CAD build for the part. Positions are in the model's coordinates, mm. Give positions to 0.01 mm unless a question says otherwise; leave off trailing zeros. Order: outer loops, then holes, each group sorted by start corner. A loop starts at its lowest first (then second) coordinate and runs counter-clockwise, first axis right, second up.
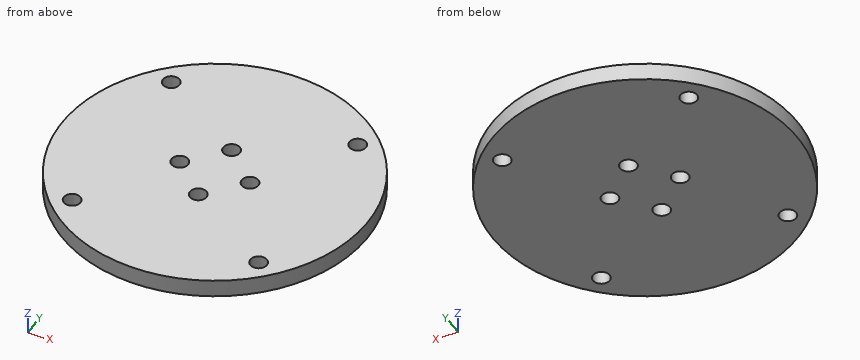
Solid Edge part; units mm, degrees
sketch "Sketch1" plane through (0, 0, 0) normal (0, 0, 1) x (1, 0, 0)
  circle A0 centre (0, 0) radius 31.0025
  circle A1 centre (19.0229, 19.0229) radius 1.7
  circle A2 centre (19.0229, -19.0229) radius 1.7
  circle A3 centre (-19.0229, -19.0229) radius 1.7
  circle A4 centre (-19.0229, 19.0229) radius 1.7
  circle A5 centre (-0.3206, 6.9927) radius 1.7
  circle A6 centre (6.9927, 0.3206) radius 1.7
  circle A7 centre (0.3206, -6.9927) radius 1.7
  circle A8 centre (-6.9927, -0.3206) radius 1.7
extrude "Protrusion1" add sketch "Sketch1" along normal blind 3.6
1. Saw through at C-C on z = 2.6. State how many separate pieces and enclosed holes the cut face has, plus the area to 3 significant figures.
2. Saw through at B-B on x = 0. Give the cut face in (y, z).
3. Wall check: line 1 (X direction, y = 1, z = 0.75); line 2 (X direction, y = -18, z = 3); line 3 (Y direction, x = 18.5, z = 1.7). Give the ranges that are in metal, low to high.
4. Saw through at A-A on x = -7. Give the cut face in (y, z).
5. Pin check, flat tips, straight feed: P1, Ø2, axis at x = 0.32, y = -6.99, coming from the +Z side; P2, Ø1, axis at x = 0.5, z = 1, coming from the +Y side. Stop position of each tip, or through.
6. Saw through at D-D on y = 25.5. Give the cut face in (x, z).
Reported:
1. separate pieces: 1
1. enclosed holes: 8
1. area: 2,950 mm2
2. outline: (-31, 0) - (-8.66, 0) - (-8.66, 3.6) - (-31, 3.6) - close; (-5.32, 0) - (5.32, 0) - (5.32, 3.6) - (-5.32, 3.6) - close; (8.66, 0) - (31, 0) - (31, 3.6) - (8.66, 3.6) - close
3. line 1: x = -30.99 to -8.06, -5.92 to 5.43, 8.55 to 30.99
3. line 2: x = -25.24 to -20.38, -17.67 to 17.67, 20.38 to 25.24
3. line 3: y = -24.88 to -20.64, -17.41 to 17.41, 20.64 to 24.88
4. outline: (-30.2, 0) - (-2.02, 0) - (-2.02, 3.6) - (-30.2, 3.6) - close; (1.38, 0) - (30.2, 0) - (30.2, 3.6) - (1.38, 3.6) - close
5. P1: passes through
5. P2: stops at y = 31
6. outline: (-17.63, 0) - (17.63, 0) - (17.63, 3.6) - (-17.63, 3.6) - close
